Can you work these out from the drawing? Everything is in mm from the part's minimum corner. A direction names the side the tool comes from. Coordinates: 2 decimals unless noted, no trailing zeros. Order: outer loops, then holes, each group sorted by start corner. A loop starts at its lowest first (then second) coordinate and runs counter-clockwise, first axis right, second up. Notation, with made-up numbers: (16, 56.25) -> (61, 56.25) arc R7 cw to (61, 62.25) -> close; hole circle Ø7 at (78.5, -31.5). An arc over 180 degrees is marked (long way). Answer in a Markdown table with one row per item.
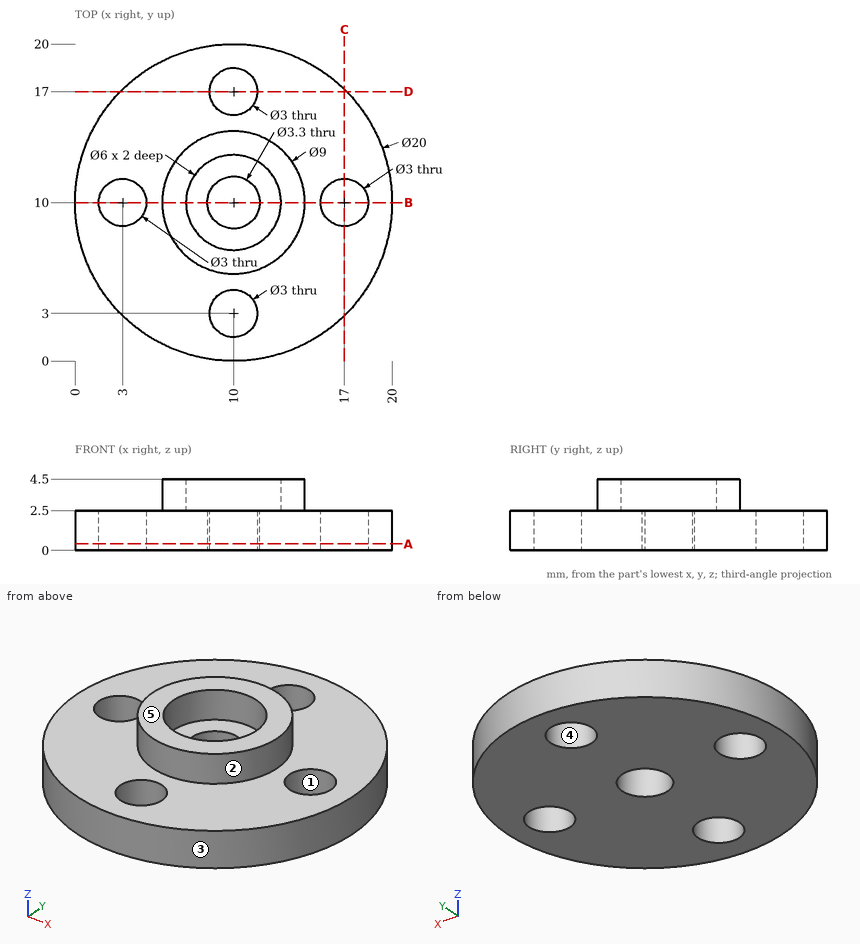
(1) We'd pull the mould along Y, two halves only. Please class the marked faces 3, 4 and 5: +Y half, -Y half, draft (parallel to the pull), parting line (faces both ways), or undercut.
Response values:
| item | result |
|---|---|
| face 3 | parting line |
| face 4 | undercut |
| face 5 | draft |
(2) I need wall thicknesses on line 1 (Y direction, x = 10, z = 1.1); line 2 (Z direction, x = 15, y = 7.25); line 3 (X direction, y = 2, z = 1.15). Which ranges of each line are inside material? Lowest first, please. Write a range as [from, to].
Response values:
| item | result |
|---|---|
| line 1 | [0, 1.5], [4.5, 8.35], [11.65, 15.5], [18.5, 20] |
| line 2 | [0, 2.5] |
| line 3 | [4, 8.88], [11.12, 16] |
(3) Suppose I cut it at C-C (x = 17). Please give me the cut outline in (y, z), and give its area (3 significant figures).
Response values:
| item | result |
|---|---|
| outline | (2.86, 0) -> (8.5, 0) -> (8.5, 2.5) -> (2.86, 2.5) -> close; (11.5, 0) -> (17.14, 0) -> (17.14, 2.5) -> (11.5, 2.5) -> close |
| area | 28.2 mm2 |
(4) On a 3-axis mill with a long thin cutter (end or side, diameter ignored), from which of +Z, -Z, +X, -X, +Y, -Y can I reach the whole of each face in a straight line? I mean the marked faces 1 and 2. Say none if no direction works.
Response values:
| item | result |
|---|---|
| face 1 | +Z, -Z |
| face 2 | +Z |
(5) Will these pins go through, and if not, where does the flat tip stop? pin 1 Ø2.5 at (x, y) = (10, 3) entering from -Z; pin 2 Ø3.5 at (x, y) = (10, 10) entering from +Z.
Response values:
| item | result |
|---|---|
| pin 1 | through |
| pin 2 | z = 2.5 |
(6) Suppose I cut it at B-B (y = 10). Please give me the cut outline in (x, z), and give its area (4 significant figures).
Response values:
| item | result |
|---|---|
| outline | (0, 0) -> (1.5, 0) -> (1.5, 2.5) -> (0, 2.5) -> close; (4.5, 0) -> (8.35, 0) -> (8.35, 2.5) -> (7, 2.5) -> (7, 4.5) -> (5.5, 4.5) -> (5.5, 2.5) -> (4.5, 2.5) -> close; (11.65, 0) -> (15.5, 0) -> (15.5, 2.5) -> (14.5, 2.5) -> (14.5, 4.5) -> (13, 4.5) -> (13, 2.5) -> (11.65, 2.5) -> close; (18.5, 0) -> (20, 0) -> (20, 2.5) -> (18.5, 2.5) -> close |
| area | 32.75 mm2 |
(7) Suppose I cut it at A-A (z = 0.4). Please give me the cut outline in (x, y), and give its area (3 significant figures).
Response values:
| item | result |
|---|---|
| outline | circle Ø20 at (10, 10); hole circle Ø3 at (3, 10); hole circle Ø3.3 at (10, 10); hole circle Ø3 at (10, 3); hole circle Ø3 at (10, 17); hole circle Ø3 at (17, 10) |
| area | 277 mm2 |
